Verification items for the finished model (mm, model axes). A direction names the side the tool comes from. Give positions to 0.01 mm unless a question says otherwise; leave off trailing zeros. Order: outer loops, then holes, each group sorted by start corner. A loop starts at its lowest first (then second) coordinate and runs counter-clockwise, first axis right, second up. Notation, with made-up numbers: (-21.75, 68) - (-9.75, 68) arc R17 cw to (-9.75, 72) - close; hole circle Ø4 at (-33.5, 34.5). An arc over 180 degrees is marked (long way). Answer as a JSON object with one key per item and string values. Group by question number.
(1) Depth check by flat-ended pin: pin 1 Ø2.5 at (x, y) = (23.55, 17.7) entering from -Z; pin 2 Ø1.5 at (x, z) = (-2.5, 0.5) entering from +Y; pin 3 Ø1.1 at (y, z) = (38.5, 2) entering from -X. Enter the tip coordinate at first touch or a pass-through.
(2) Thickness scan on line 1 (X direction, y = -10, z = 1.75); line 2 (X direction, y = 68.1, z = 2.1); line 3 (Y direction, x = 17.5, z = 2.25). Record the ranges inside material, lowest first.
(3) Access from +Z, -Z, +X, -X, +Y, -Y to the whole of each face (thin tool, end or side, straight path). Record for faces 1 (the face through (42.35, 0, 2)), 2 (the face through (28.75, 63.62, 1.87)), 3 (the face through (-3, 13.5, 2)), 4 (the face through (38, 13.5, 2)).
(4) Section check D-D (x = 36.5). Record the boundary of the cut face in (y, z), then the cut area to 3 significant figures.
(5) Section check B-B (y = 17.7). Record the boundary of the cut face in (x, z).
(6) Mould release check, pull along Y, two halves, no side actions. Record for faces 5 (the face through (22, 17, 2)), 6 (the face through (18, 20, 0)), 7 (the face through (33.1, 69.73, 1.87)): +Y half, -Y half, draft (parallel to the pull), parting line (faces both ways), or undercut.
(7) Section check A-A (y = 32). Record the boundary of the cut face in (x, z), then the cut area to 3 significant figures.
(8) Section check C-C (z = 1.4). Count the separate pieces of the cut face and the enclosed holes in it, then the cut area to 3 significant figures.
```python
from build123d import *

# Parameters (mm, degrees)
SKETCH1_R           = 1.7
BOSS_EXTRUDE1_DEPTH = 3.8


with BuildPart() as part:
    # Sketch1 → Boss-Extrude1 (new body)
    with BuildSketch(Plane.XY):
        with BuildLine():
            Line((3.000019473, 70.3), (31.700019473, 70.3))
            ThreePointArc((31.700019473, 70.3), (33.114233035, 69.714213562), (33.700019473, 68.3))
            Line((33.700019473, 68.3), (33.700019473, 15.5))
            ThreePointArc((33.700019473, 15.5), (34.285805911, 14.085786438), (35.700019473, 13.5))
            Line((35.700019473, 13.5), (40.350019473, 13.5))
            ThreePointArc((40.350019473, 13.5), (41.764233035, 12.914213562), (42.350019473, 11.5))
            Line((42.350019473, 11.5), (42.350019473, -11.641128199))
            ThreePointArc((42.350019473, -11.641128199), (41.764233035, -13.055341761), (40.350019473, -13.641128199))
            Line((40.350019473, -13.641128199), (31.700019473, -13.641128199))
            Line((31.700019473, -13.641128199), (3.000019473, -13.641128199))
            Line((3.000019473, -13.641128199), (-5.649980527, -13.641128199))
            ThreePointArc((-5.649980527, -13.641128199), (-7.064194089, -13.055341761), (-7.649980527, -11.641128199))
            Line((-7.649980527, -11.641128199), (-7.649980527, 11.5))
            ThreePointArc((-7.649980527, 11.5), (-7.064194089, 12.914213562), (-5.649980527, 13.5))
            Line((-5.649980527, 13.5), (-0.999980527, 13.5))
            ThreePointArc((-0.999980527, 13.5), (0.414233035, 14.085786438), (1.000019473, 15.5))
            Line((1.000019473, 15.5), (1.000019473, 68.3))
            ThreePointArc((1.000019473, 68.3), (1.585805911, 69.714213562), (3.000019473, 70.3))
        make_face()
        with Locations(Location((11.15, 17.7, 0), (0, 0, 180))):
            Circle(SKETCH1_R, mode=Mode.SUBTRACT)
        with Locations(Location((9.85, 10, 0), (0, 0, 180))):
            Circle(SKETCH1_R, mode=Mode.SUBTRACT)
        with Locations(Location((24.85, 10, 0), (0, 0, 180))):
            Circle(SKETCH1_R, mode=Mode.SUBTRACT)
        with Locations(Location((9.85, -10, 0), (0, 0, 180))):
            Circle(SKETCH1_R, mode=Mode.SUBTRACT)
        with Locations(Location((24.85, -10, 0), (0, 0, 180))):
            Circle(SKETCH1_R, mode=Mode.SUBTRACT)
        with Locations(Location((23.55, 17.7, 0), (0, 0, 180))):
            Circle(SKETCH1_R, mode=Mode.SUBTRACT)
        with Locations(Location((23.55, 68.1, 0), (0, 0, 180))):
            Circle(SKETCH1_R, mode=Mode.SUBTRACT)
        with Locations(Location((11.15, 68.1, 0), (0, 0, 180))):
            Circle(SKETCH1_R, mode=Mode.SUBTRACT)
        with BuildLine():
            Line((7.35, 64.190811085), (27.35, 64.190811085))
            ThreePointArc((27.35, 64.190811085), (28.764213562, 63.605024648), (29.35, 62.190811085))
            Line((29.35, 62.190811085), (29.35, 23.654008347))
            ThreePointArc((29.35, 23.654008347), (28.764213562, 22.239794784), (27.35, 21.654008347))
            Line((27.35, 21.654008347), (7.35, 21.654008347))
            ThreePointArc((7.35, 21.654008347), (5.935786438, 22.239794784), (5.35, 23.654008347))
            Line((5.35, 23.654008347), (5.35, 62.190811085))
            ThreePointArc((5.35, 62.190811085), (5.935786438, 63.605024648), (7.35, 64.190811085))
        make_face(mode=Mode.SUBTRACT)
    extrude(amount=BOSS_EXTRUDE1_DEPTH)


solid = part.part
```
Solutions:
{
 "1": {"pin 1": "passes through", "pin 2": "stops at y = 13.5", "pin 3": "stops at x = 1"},
 "2": {"line 1": "x = -7.65 to 8.15, 11.55 to 23.15, 26.55 to 42.35", "line 2": "x = 1 to 9.45, 12.85 to 21.85, 25.25 to 33.7", "line 3": "y = -13.64 to 21.65, 64.19 to 70.3"},
 "3": {"face 1": "+Z, -Z, +X, +Y, -Y", "face 2": "+Z, -Z", "face 3": "+Z, -Z, -X, +Y", "face 4": "+Z, -Z, +X, +Y"},
 "4": {"outline": "(-13.64, 0) - (13.5, 0) - (13.5, 3.8) - (-13.64, 3.8) - close", "area": "103 mm2"},
 "5": {"outline": "(1, 0) - (9.45, 0) - (9.45, 3.8) - (1, 3.8) - close; (12.85, 0) - (21.85, 0) - (21.85, 3.8) - (12.85, 3.8) - close; (25.25, 0) - (33.7, 0) - (33.7, 3.8) - (25.25, 3.8) - close"},
 "6": {"face 5": "undercut", "face 6": "draft", "face 7": "+Y half"},
 "7": {"outline": "(1, 0) - (5.35, 0) - (5.35, 3.8) - (1, 3.8) - close; (29.35, 0) - (33.7, 0) - (33.7, 3.8) - (29.35, 3.8) - close", "area": "33.1 mm2"},
 "8": {"separate pieces": "1", "enclosed holes": "9", "area": "2,120 mm2"}
}
